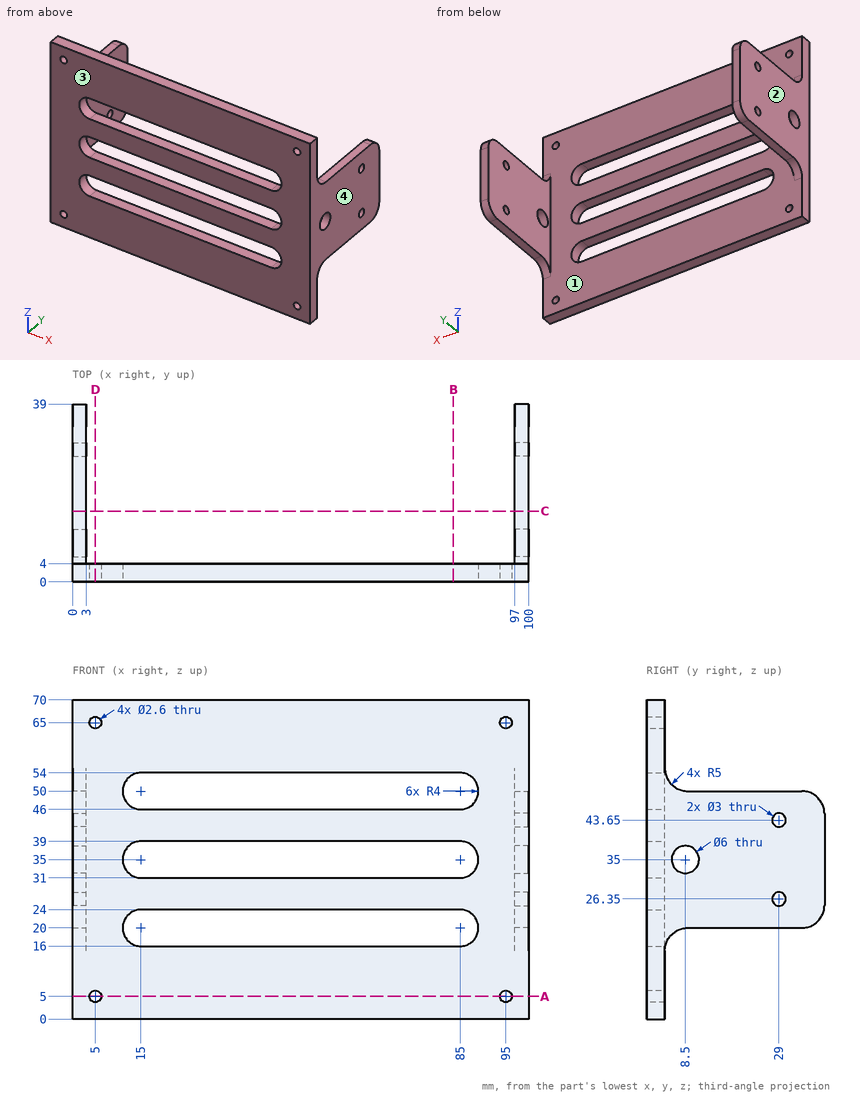
Study the drawing (mm; zero at the part's minimum x, y, z) and answer. Round coordinates to 2 decimals unless told otherwise and drop trailing zeros. Order: outer loops, then holes, each group sorted by start corner. A loop starts at its lowest first (then second) coordinate and runs counter-clockwise, first axis right, second up. Notation, with made-up numbers: (39.5, 32.25) - (98.5, 32.25) arc R14 cw to (98.5, 56.25) - close; hole circle Ø10 at (45.25, 3). An arc over 180 degrees is marked (long way). Use one line per item in the form item = value. Start each with the question number.
(1) Determine the mould class of the marked faces 1, 2, 3 and 4 for opening direction X: +X half, -X half, draft (parallel to the pull), parting line (faces both ways), or undercut.
(2) Flat-ended cylindrical pins translate along their axes: pin 1 Ø4 at (x, z) = (80.5, 31.5) entering from +Y; pin 2 Ø3.5 at (x, y) = (1.5, 16) entering from -Z; pin 3 Ø0.9 at (x, y) = (99, 22.5) entering from +Z. Find the tip coordinate at first contact, or state that the pin passes through.
(3) The part is cut by section D-D (x = 5). Give the vertices of the cut face in (y, z).
(4) Find the intervals of material crossed by line 1 along X through (y, z) = (2.9, 65); line 2 along Z through (x, y) = (95, 1.45); line 3 along Y through (x, z) = (97.6, 26.35), in increasing order. Write a range as from..to.
(5) The part is cut by section B-B (x = 83.5). Give the vertices of the cut face in (y, z), then the cut area to 3 significant figures.
(6) The part is cut by section A-A (z = 5). Give the vertices of the cut face in (x, y), then the cut area to 3 significant figures.
(7) The part is cut by section C-C (y = 15.5). Give the vertices of the cut face in (x, z).
Checked values:
q1.face_1 = undercut
q1.face_2 = -X half
q1.face_3 = draft
q1.face_4 = +X half
q2.pin_1 = 4
q2.pin_2 = 20
q2.pin_3 = 50
q3.outline = (0, 0) - (4, 0) - (4, 3.7) - (0, 3.7) - close; (0, 6.3) - (4, 6.3) - (4, 63.7) - (0, 63.7) - close; (0, 66.3) - (4, 66.3) - (4, 70) - (0, 70) - close
q4.line_1 = 0..3.7, 6.3..93.7, 96.3..100
q4.line_2 = 0..3.7, 6.3..63.7, 66.3..70
q4.line_3 = 0..27.5, 30.5..39
q5.outline = (0, 0) - (4, 0) - (4, 16) - (0, 16) - close; (0, 24) - (4, 24) - (4, 31) - (0, 31) - close; (0, 39) - (4, 39) - (4, 46) - (0, 46) - close; (0, 54) - (4, 54) - (4, 70) - (0, 70) - close
q5.area = 184 mm^2
q6.outline = (0, 0) - (3.7, 0) - (3.7, 4) - (0, 4) - close; (6.3, 0) - (93.7, 0) - (93.7, 4) - (6.3, 4) - close; (96.3, 0) - (100, 0) - (100, 4) - (96.3, 4) - close
q6.area = 379 mm^2
q7.outline = (0, 20) - (3, 20) - (3, 50) - (0, 50) - close; (97, 20) - (100, 20) - (100, 50) - (97, 50) - close
